```python
from build123d import *

# Parameters (mm, degrees)
SWEEP_THIN1_PROFILE_R   = 30
SWEEP_THIN1_PROFILE_R_2 = 20
CUT_EXTRUDE1_DEPTH      = 1315.343942812
CUT_EXTRUDE1_DEPTH_BACK = 1315.343942812
SKETCH18_R              = 20
SKETCH19_R              = 20
CUT_EXTRUDE2_DEPTH      = 100


with BuildPart() as part:
    # Sweep-Thin1: sweep along a path in Sketch1
    with BuildLine(Plane(origin=(0, 0, 0), x_dir=(0, 0, -1), z_dir=(1, 0, 0))) as sweep_thin1_path:
        Line((0, 0), (150, 0))
        ThreePointArc((150, 0), (220.710678119, -29.289321881), (250, -100))
        Line((250, -100), (250, -760))
        Line((250, -760), (1050, -760))
    # Sweep-Thin1 profile (on start of the path) → Sweep-Thin1 (sweep)
    with BuildSketch(Plane(origin=(0, 0, 0), x_dir=(-1, 0, 0), z_dir=(0, 0, -1))):
        Circle(SWEEP_THIN1_PROFILE_R)
        Circle(SWEEP_THIN1_PROFILE_R_2, mode=Mode.SUBTRACT)
    sweep(path=sweep_thin1_path.line, transition=Transition.RIGHT)

    # Sketch18 → Cut-Extrude1 (cut, two sides: drawn at the far end of the back side and taken through both)
    with BuildSketch(Plane(origin=(0, 0, 0), x_dir=(0, 0, -1), z_dir=(1, 0, 0)).offset(-CUT_EXTRUDE1_DEPTH_BACK)):
        with Locations(Location((250, -760, 0), (0, 0, 315.000007379))):
            Circle(SKETCH18_R)
    extrude(amount=CUT_EXTRUDE1_DEPTH + CUT_EXTRUDE1_DEPTH_BACK, mode=Mode.SUBTRACT)

    # Sketch19 → Cut-Extrude2 (cut)
    with BuildSketch(Plane.XY.offset(-350)):
        with Locations(Location((0, -285, 0), (0, 0, 270))):
            Circle(SKETCH19_R)
    extrude(amount=CUT_EXTRUDE2_DEPTH, mode=Mode.SUBTRACT)


solid = part.part
```
Geometry check sheet. Reference: the model listing, model coordinates, mm. A direction names the side the tool comes from. Round coordinates to 2 decimals unless told otherwise and drop trailing zeros. Order: outer loops, then holes, each group sorted by start corner. A loop starts at its lowest first (then second) coordinate and runs counter-clockwise, first axis right, second up. Notation, with made-up numbers: (-31.75, 46) -> (4.25, 46) arc R22 cw to (4.25, 67) -> close; hole circle Ø7 at (24, 78.5). An arc over 180 degrees is marked (long way). Return JSON: item names as keys, results as strings. Group by question number.
Q1. Section check A-A, the plane z = -962.5. Record the boundary of the cut face in (x, y), plus the area to 3 significant figures.
Q2. Tool access check on faces 5 (the cylindrical face through (18.12, -770.74, -233.13)), 6 (the cylindrical face through (4.336, -434.62, -230.476)), 7 (the cylindrical face through (16.864, -295.752, -268.543)), 8 (the cylindrical face through (29.97, 1.32, -76.05)). Record the directions out of +Z, -Z, +X, -X, +Y, -Y that give a thin tool (end or side, any length) a straight path to the whole face; none if there is none.
Q3. Material ranges on probe 1 along Y at (x, z) = (0, -102); probe 2 along Y at (x, z) = (-2, -711); probe 3 along Z at (x, y) = (-1, -127), recorded low to high. Write a range as from..to.
Q4. Release check for a two-part mould opening along Z. For faces 1 (the flat face through (-6, -780, -1050)), 2 (the cylindrical face through (6.503, -449.83, -220.713)), 3 (the cylindrical face through (-18.54, -770.74, -233.13)), 4 (the cylindrical face through (6.503, -789.287, -640.81)) record: released by +Z, released by -Z, zero draft, split by the parting line, or undercut.
Q5. Gauge pin test, flat ends, axial feed: pin 1 (24 mm diameter, centred on x = 0, z = -250, fed in from +Y); pin 2 (5 mm diameter, centred on x = -12, y = -472.5, fed in from +Z); pin 3 (6 mm diameter, centred on x = -3.5, y = -115.5, fed in from +Z). Record the tip position at first contact, or that the pin passes through.
Q6. Section check B-B, the plane y = -529.5. Record the boundary of the cut face in (x, z).
Numbers:
{
 "1": {"outline": "circle Ø60 at (0, -760); hole circle Ø40 at (0, -760)", "area": "1,570 mm^2"},
 "2": {"face 5": "+X, -X", "face 6": "none", "face 7": "-Z", "face 8": "+Z"},
 "3": {"probe 1": "-30..-20, 20..30", "probe 2": "-789.93..-779.9, -740.1..-730.07", "probe 3": "-279.98..-269.97, -230.03..-220.02"},
 "4": {"face 1": "released by -Z", "face 2": "split by the parting line", "face 3": "undercut", "face 4": "zero draft"},
 "5": {"pin 1": "y = -4.31", "pin 2": "z = -221.54", "pin 3": "z = -220"},
 "6": {"outline": "circle Ø60 at (0, -250); hole circle Ø40 at (0, -250)"}
}
